Input: part model. Units: mm. Frame: model coordinates. Face numbers are marked on the shaded views. Give positions to 0.01 mm unless a question says otherwise; leave off trailing zeros. Loops run counter-clockwise (first coordinate to the right, second up) from the corner with the lowest first, then second, coordinate; pieces in that order, holes last. Notation, with made-up numbers: M 83,32 L 95,32 A8 cw 95,44 Z; hole C 27,-2 d11. An arc over 180 degrees is marked long. Return JSON: item names as keys, results as strings. Group by question number.
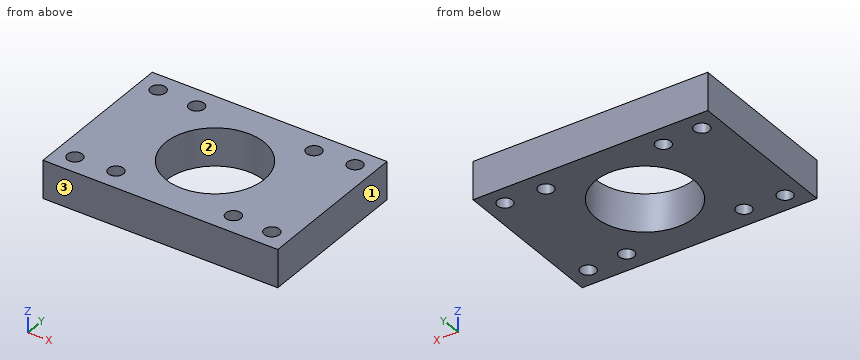
Autodesk Inventor part; units mm, degrees
ref_plane "YZ Plane" through (0, 0, 0) normal (1, 0, 0) x (0, 1, 0)
ref_plane "XZ Plane" through (0, 0, 0) normal (0, 1, 0) x (-1, 0, 0)
ref_plane "XY Plane" through (0, 0, 0) normal (0, 0, 1) x (1, 0, 0)
sketch "Sketch1" plane through (0, 0, 0) normal (0, 0, 1) x (1, 0, 0)
  line L0 (0, 0) -> (0, -42)
  line L1 (0, -42) -> (62, -42)
  line L2 (62, -42) -> (62, 0)
  line L3 (62, 0) -> (0, 0)
  line L4 (11, -42) -> (53, -42)
  line L5 (53, 0) -> (11, 0)
  line L6 (10, -5.9896) -> (10, -30.0104)
  line L7 (31, 0) -> (31, -13)
  circle A0 centre (5, -5) radius 2
  line L8 (0, -21) -> (-21.0238, -21)
  circle A1 centre (31, -21) radius 13
  circle A2 centre (15.5, -5.5) radius 2
  circle A3 centre (15.5, -36.5) radius 2
  circle A4 centre (5, -37) radius 2
  line L9 (52, -5.9896) -> (52, -30.0104)
  circle A5 centre (57, -5) radius 2
  circle A6 centre (46.5, -5.5) radius 2
  circle A7 centre (46.5, -36.5) radius 2
  circle A8 centre (57, -37) radius 2
  dimension "d0" = 42
  dimension "d1" = 62
  dimension "d42" = 10
  dimension "d43" = 4
  dimension "d44" = 5
  dimension "d45" = 5
  dimension "d46" = 26
  dimension "d47" = 4
  dimension "d50" = 4
  dimension "d51" = 5.5
  dimension "d52" = 5.5
  dimension "d53" = 5.5
  dimension "d54" = 31
extrude "Extrusion4" add sketch "Sketch1" along normal blind 10
thread "Rosca1"
thread "Rosca2"
thread "Rosca3"
thread "Rosca4"
properties part number "Techo Espaciador Sub. Inferior" material "Aluminum 6061"
Item 1: First-contact query: pin 1 Ø2.5 at (x, y) = (57, -5) entering from +Z. Flat tip, straight axial feed; report the tip coordinate or a pass-through.
Item 2: Section A-A, the plane y = -21. Return loops of the section in (x, z), then the cut area to 3 significant figures.
Item 3: Section C-C, the plane z = 9.25. Give the number of separate pieces and of enclosed holes in the cut face, then the cut area to 3 significant figures.
Item 4: Section D-D, the plane x = 46.5. Return loops of the section in (y, z).
Item 5: Pull-direction query (Y, two-part tool) for the marked faces 1, 2 and 3; classes: pulls with the +Y half, pulls with the -Y half, needs draft (parallel to the pull), parting line crosses it, or undercut.
Item 6: Section B-B, the plane x = 31. Return loops of the section in (y, z).
Item 7: Material intervals for line 1 (Y direction, x = 57, z = 5.5); line 2 (X direction, y = -36, z = 2); line 3 (Y direction, x = 31, z = 5.25), sorted ascending. Write a range as from..to.
Answer below:
{
 "1": {"pin 1": "through"},
 "2": {"outline": "M 0,0 L 18,0 L 18,10 L 0,10 Z; M 44,0 L 62,0 L 62,10 L 44,10 Z", "area": "360 mm^2"},
 "3": {"separate pieces": "1", "enclosed holes": "9", "area": "1,970 mm^2"},
 "4": {"outline": "M -42,0 L -38.5,0 L -38.5,10 L -42,10 Z; M -34.5,0 L -7.5,0 L -7.5,10 L -34.5,10 Z; M -3.5,0 L 0,0 L 0,10 L -3.5,10 Z"},
 "5": {"face 1": "needs draft", "face 2": "undercut", "face 3": "pulls with the -Y half"},
 "6": {"outline": "M -42,0 L -34,0 L -34,10 L -42,10 Z; M -8,0 L 0,0 L 0,10 L -8,10 Z"},
 "7": {"line 1": "-42..-39, -35..-7, -3..0", "line 2": "0..3.27, 6.73..13.56, 17.44..44.56, 48.44..55.27, 58.73..62", "line 3": "-42..-34, -8..0"}
}
